Can you work these out from the model? Positions are in its coordinate system, mm. A direction names the side the tool comes from. Coordinates: 2 decimals unless noted, no trailing zeros. Order: outer loops, then holes, each group sorted by start corner. A loop starts at its lowest first (then second) coordinate and runs counter-clockwise, first axis right, second up. Notation, with made-up numbers: (37, -0.75) -> (66, -0.75) arc R5 cw to (66, 7.25) -> close; hole circle Ø5 at (28.25, 26.5). An arc over 180 degrees is marked (long way). Answer in a Markdown table with one row per item. Add a question column.
1. On a 3-axis mill with a long thin cutter (end or side, diameter ignored), from which of +Z, -Z, +X, -X, +Y, -Y can I reach the whole of each face in a straight line? I mean faces 4 (the face through (-1.2, 1.5, -0.3)), 5 (the face through (0, 3, 4)). Say none if no direction works.
2. Imagine slicing it at D-D on x = 14. Write out the boundary of the cut face in (y, z).
3. If I drill on line 1 along X through (y, z) = (1.95, -0.5); line 2 along X through (y, z) = (1.85, -5); line 3 along X through (y, z) = (2.4, -11.5), over which ranges is the centre line in solid material (lowest first)? Write a range as [from, to].
4. We'd pull the mould along Z, two halves only. Please class faces 1 (the face through (-19.524, 1.479, -4.336)), 2 (the face through (0, 0, 4)), 3 (the face through (10.05, 1.52, -0.33)): pulls with the +Z half, pulls with the -Z half, needs draft (parallel to the pull), parting line crosses it, or undercut.
5. Imagine slicing it at C-C on y = 2.1. Write out the boundary of the cut face in (x, z), plus the area to 3 significant figures.
6. Will these pins go through, and if not, where does the flat tip stop? pin 1 (1.5 mm diameter, centred on x = 12, y = 2, fed in from -Z); pin 2 (1 mm diameter, centred on x = -12, y = 2.5, fed in from +Z); pin 3 (1 mm diameter, centred on x = 11, y = 0.5, fed in from +Z).
7. Imagine slicing it at A-A on x = 0. Write out the boundary of the cut face in (y, z).
8. Imagine slicing it at B-B on z = -7. Write out the boundary of the cut face in (x, y) (3 decimals), plus the area to 3 significant figures.
from build123d import *

# Parameters (mm, degrees)
SKETCH1_R           = 20
BOSS_EXTRUDE1_DEPTH = 3
SKETCH2_W           = 3
SKETCH2_H           = 15
CUT_EXTRUDE1_DEPTH  = 3
SKETCH3_R           = 1.5
CUT_EXTRUDE2_DEPTH  = 3
FILLET1_R           = 1
FILLET2_R           = 1
FILLET3_R           = 1
FILLET4_R           = 1


with BuildPart() as part:
    # Sketch1 → Boss-Extrude1 (new body)
    with BuildSketch(Plane(origin=(0, 0, 0), x_dir=(1, 0, 0), z_dir=(0, 1, 0))):
        with Locations(Location((0, 0, 0), (0, 0, 270))):
            Circle(SKETCH1_R)
    extrude(amount=BOSS_EXTRUDE1_DEPTH)

    # Sketch2 → Cut-Extrude1 (cut)
    with BuildSketch(Plane(origin=(0, 3, 0), x_dir=(1, 0, 0), z_dir=(0, 1, 0))):
        with Locations((0.013912119, 7.5)):
            Rectangle(SKETCH2_W, SKETCH2_H)
    extrude(amount=-CUT_EXTRUDE1_DEPTH, mode=Mode.SUBTRACT)

    # Sketch3 → Cut-Extrude2 (cut)
    with BuildSketch(Plane(origin=(0, 3, 0), x_dir=(1, 0, 0), z_dir=(0, 1, 0))):
        with Locations(Location((11.513912119, 0, 0), (0, 0, 270))):
            Circle(SKETCH3_R)
    extrude(amount=-CUT_EXTRUDE2_DEPTH, mode=Mode.SUBTRACT)

    # Fillet1
    fillet1_edges = [part.edges().sort_by_distance(p)[0] for p in [
        (-1.486087881, 1.5, -15),
    ]]
    fillet(fillet1_edges, radius=FILLET1_R)

    # Fillet2
    fillet2_edges = [part.edges().sort_by_distance(p)[0] for p in [
        (1.513912119, 1.5, -15),
    ]]
    fillet(fillet2_edges, radius=FILLET2_R)

    # Fillet3
    fillet3_edges = [part.edges().sort_by_distance(p)[0] for p in [
        (-1.486087881, 1.5, 0),
    ]]
    fillet(fillet3_edges, radius=FILLET3_R)

    # Fillet4
    fillet4_edges = [part.edges().sort_by_distance(p)[0] for p in [
        (1.513912119, 1.5, 0),
    ]]
    fillet(fillet4_edges, radius=FILLET4_R)


solid = part.part
Answers follow:
| question | item | result |
|---|---|---|
| 1 | face 4 | +Y, -Y |
| 1 | face 5 | +Z, -Z, +X, -X, +Y |
| 2 | outline | (0, -14.28) -> (3, -14.28) -> (3, 14.28) -> (0, 14.28) -> close |
| 3 | line 1 | x = [-19.99, -1.35], [1.38, 10.1], [12.93, 19.99] |
| 3 | line 2 | x = [-19.36, -1.49], [1.51, 19.36] |
| 3 | line 3 | x = [-16.36, -1.49], [1.51, 16.36] |
| 4 | face 1 | parting line crosses it |
| 4 | face 2 | needs draft |
| 4 | face 3 | undercut |
| 5 | outline | circle Ø40 at (0, 0); hole (-1.49, -14) arc R1 ccw to (-0.49, -15) -> (0.51, -15) arc R1 ccw to (1.51, -14) -> (1.51, -1) arc R1 ccw to (0.51, 0) -> (-0.49, 0) arc R1 ccw to (-1.49, -1) -> close; hole circle Ø3 at (11.51, 0) |
| 5 | area | 1,210 mm² |
| 6 | pin 1 | stops at z = -16.54 |
| 6 | pin 2 | stops at z = 16.36 |
| 6 | pin 3 | stops at z = 17.02 |
| 7 | outline | (0, -20) -> (3, -20) -> (3, -15) -> (0, -15) -> close; (0, 0) -> (3, 0) -> (3, 20) -> (0, 20) -> close |
| 8 | outline | (-18.735, 0) -> (-1.486, 0) -> (-1.486, 3) -> (-18.735, 3) -> close; (1.514, 0) -> (18.735, 0) -> (18.735, 3) -> (1.514, 3) -> close |
| 8 | area | 103 mm² |
